Autodesk Inventor part; units mm, degrees
ref_plane "YZ Plane" through (0, 0, 0) normal (1, 0, 0) x (0, 1, 0)
ref_plane "XZ Plane" through (0, 0, 0) normal (0, 1, 0) x (-1, 0, 0)
ref_plane "XY Plane" through (0, 0, 0) normal (0, 0, 1) x (1, 0, 0)
sketch "Szkic1" plane through (0, 0, 0) normal (0, 1, 0) x (-1, 0, 0)
  line L0 (28, 0) -> (0, 0)
  line L1 (0, 0) -> (0, -8)
  line L2 (0, -8) -> (28, -8)
  line L3 (28, -8) -> (28, 0)
  dimension "d0" = 8
  dimension "d4" = 28
extrude "Wyciągnięcie proste1" add sketch "Szkic1" along normal blind 2.5
sketch "Szkic2" plane through (0, 2.5, 0) normal (0, 1, 0) x (1, 0, 0)
  line L0 (-28, 0) -> (0, 0)
  line L1 (0, 8) -> (-28, 8)
  line L2 (-14, 0) -> (-14, 8)
  line L3 (-24, 4) -> (-4, 4)
  point P0 (-14, 4)
  dimension "d3" = 20
hole "Otwór1" at (-24, 2.5, -4) at (-4, 2.5, -4) direction (0, -1, 0) diameter 2.6 end through all counterbore diameter 4.5 counterbore depth 1.5
sketch "Szkic3" plane through (-28, 0, 0) normal (0, 0, 1) x (1, 0, 0)
  line L0 (14, 2.5) -> (14, 0)
  line L1 (0, 2.5) -> (28, 2.5)
  line L2 (0, 0) -> (28, 0)
  circle A0 centre (14, -5) radius 2.5
  line L3 (10, -5) -> (18, -5)
  line L4 (18, -5) -> (18, 0)
  line L5 (10, 0) -> (10, -5)
  line L6 (18, 0) -> (10, 0)
  point P0 (10, 3)
  point P1 (17.6174, 3)
  point P2 (16.5, -5)
  point P3 (11.5, -5)
  point P4 (14, 0)
  point P5 (18, 0)
  dimension "d12" = 5
  dimension "d13" = 8
  dimension "d17" = 5
extrude "Wyciągnięcie proste2" add sketch "Szkic3" against normal up to surface (8 mm away) contours L2 L4 L3 A0 L5
fillet "Zaokrąglenie1" radius 2 4 edges at (0, 1.25, 0) (0, 1.25, -8) (-28, 1.25, -8) (-28, 1.25, 0)
equation "\"d0\" = obudowa_led_mocowanie_grubosc"
equation "\"d4\" = holder_led_dlugosc"
equation "\"d1\" = holder_led_grubosc"
equation "\"d5\" = gniazdo_M2_D2"
equation "\"d7\" = gniazdo_M2_D1"
equation "\"d8\" = gniazdo_M2_glebokosc"
equation "\"d10\" = insert_glebokosc"
equation "\"d12\" = holder_led_uchwyt_D"
equation "\"d13\" = holder_led_uchwyt_szerokosc"
equation "\"d17\" = holder_led_uchwyt_wysokosc"
equation "\"gniazdo_M2_glebokosc\" = 1.5"
equation "\"gniazdo_M2_D1\" = 4.5"
equation "\"gniazdo_M2_D2\" = 2.6"
equation "\"insert_D\" = 2.9"
equation "\"insert_glebokosc\" = 7"
equation "\"podstawa_wys\" = 2"
equation "\"podstawa_otwory_montazowe_poz_x\" = 4"
equation "\"podstawa_otwory_montazowe_poz_y\" = 4"
equation "\"podstawa_zaokraglenie\" = 3"
equation "\"obudowa_wys\" = 45"
equation "\"obudowa_grubosc\" = 2"
equation "\"obudowa_kontrolki_a\" = 38"
equation "\"obudowa_otwory_montazowe_poz_x\" = 4"
equation "\"obudowa_otwory_montazowe_poz_y\" = 4"
equation "\"obudowa_otwory_montazowe_material_x\" = 8"
equation "\"obudowa_otwory_montazowe_material_y\" = 8"
equation "\"obudowa_zaokraglenie\" = 3"
equation "\"obudowa_otwory_io1_D\" = 12"
equation "\"obudowa_otwory_io1_wys\" = 25"
equation "\"obudowa_otwory_io1_poz\" = 55"
equation "\"obudowa_otwory_io2_D\" = 12"
equation "\"obudowa_otwory_io2_wys\" = 25"
equation "\"obudowa_otwory_io2_poz\" = 38"
equation "\"obudowa_otwory_pot_D\" = 7.2"
equation "\"obudowa_pot_poz_y\" = 15"
equation "\"obudowa_s_rozstaw_y\" = 16"
equation "\"obudowa_s_poz_x\" = 78"
equation "\"obudowa_s_poz_y\" = 15"
equation "\"obudowa_s_D\" = 6.2"
equation "\"input_a\" = 8.9"
equation "\"input_b\" = 14.4"
equation "\"input_wys\" = 10.9"
equation "\"obudowa_MTS_otwor_D\" = 6.2"
equation "\"pcb_rozstaw_x\" = 92"
equation "\"pcb_rozstaw_y\" = 58"
equation "\"pcb_grubosc_scianki\" = 6"
equation "\"pcb_wys_bloku\" = 35"
equation "\"pcb_poz_y\" = 29"
equation "\"obudowa_footswitch_D\" = 12.3"
equation "\"obudowa_footswitch_poz_x\" = 35"
equation "\"obudowa_footswitch_poz_y\" = 68"
equation "\"obudowa_led_indicator_D\" = 3.5"
equation "\"obudowa_led_indicator_poz_x\" = 55"
equation "\"obudowa_podkladka_otwory\" = 4"
equation "\"obudowa_uchwyt_poz_z\" = 3"
equation "\"obudowa_uchwyt_grubosc\" = 2"
equation "\"obudowa_uchwyt_szerokosc_wew\" = 17.5"
equation "\"obudowa_uchwyt_wysokosc_wew\" = 26.3"
equation "\"obudowa_uchwyt_kolnierz_wys\" = 55"
equation "\"obudowa_gniazdo_poz\" = 25"
equation "\"obudowa_podciecie_inout_wys\" = 6"
equation "\"obudowa_podciecie_logo_wys\" = 34"
equation "\"obudowa_podciecie_logo_szerokosc\" = 25"
equation "\"obudowa_pot_pozycjonowanie_szerokosc\" = 2.8"
equation "\"obudowa_pot_pozycjonowanie_wys\" = 13"
equation "\"obudowa_pot_pozycjonowanie_glebokosc\" = 1.4"
equation "\"obudowa_led_mocowanie_wys\" = 6"
equation "\"obudowa_led_mocowanie_grubosc\" = 8"
equation "\"obudowa_led_mocowanie_rozstaw_otworow\" = 20"
equation "\"holder_led_grubosc\" = 2.5"
equation "\"holder_led_dlugosc\" = 28"
equation "\"holder_led_uchwyt_D\" = 5"
equation "\"holder_led_uchwyt_wysokosc\" = 5"
equation "\"holder_led_uchwyt_szerokosc\" = 8"
equation "\"holder_gniazdo_b\" = 5"
equation "\"holder_gniazdo_grubosc\" = 2.5"
equation "\"holder_gniazdo_a\" = 28"
equation "\"podstawa_mocowanie_DC_a\" = 7"
equation "\"podstawa_mocowanie_DC_b\" = 8.9"
equation "\"podstawa_mocowanie_DC_wys\" = 6"
equation "\"holder_gniazdo_odleglosc_miedzy_ramionami\" = 9.2"
equation "\"holder_gniazdo_grubosc_ramion\" = 1.5"
equation "\"holder_gniazdo_wys\" = 8"
equation "\"holder_gniazdo_uchwyt_poz\" = 5"
properties part number "led_holder"
Here's how the part is built. I have some questions about the finished solid (model axes, mm). A direction names the side the tool comes from. Round coordinates to 2 decimals unless told otherwise and drop trailing zeros. Loops run counter-clockwise (first coordinate to the right, second up) from the corner with the lowest first, then second, coordinate; pieces in that order, holes last. Notation, with made-up numbers: (-17.75, -14.5) -> (31.25, -14.5) arc R24 ccw to (31.25, 20.5) -> close; hole circle Ø11 at (44.5, -34.5). An arc over 180 degrees is marked (long way). Write each question's results on one line, items separated by ' | '.
(1) If we section it at B-B, the plane x = -24: List the corners of the cut face in (y, z) for me.
Worked answers:
outline: (0, -8) -> (2.5, -8) -> (2.5, -6.25) -> (1, -6.25) -> (1, -5.3) -> (0, -5.3) -> close; (0, -2.7) -> (1, -2.7) -> (1, -1.75) -> (2.5, -1.75) -> (2.5, 0) -> (0, 0) -> close
(2) If we section it at A-A, the plane y = -3.5: List the corners of the cut face in (x, z) for me, then the cut area to 3 significant figures.
Worked answers:
outline: (-18, -8) -> (-16, -8) -> (-16, 0) -> (-18, 0) -> close; (-12, -8) -> (-10, -8) -> (-10, 0) -> (-12, 0) -> close | area: 32.0 mm2
(3) If I drill on L1, parallel to X at y = 2.05, z = -4; L2, parallel to X at y = 0.45, z = -4; L3, parallel to Z at x = -24, y = 0.65, over which ranges is the centre line in solid material (lowest first)?
Worked answers:
L1: -28 to -26.25, -21.75 to -6.25, -1.75 to 0 | L2: -28 to -25.3, -22.7 to -5.3, -2.7 to 0 | L3: -8 to -5.3, -2.7 to 0
(4) We'd pull the mould along X, two halves only. Please class faces 4 (the face through (-13.9, -2.5, -3.9)), 5 (the face through (-14, 0, -8)), 6 (the face through (-27.43, 1.27, -0.6)), 7 (the face through (-0.57, 1.27, -7.4)): released by +X, released by -X, zero draft, split by the parting line, or undercut.
Worked answers:
face 4: undercut | face 5: zero draft | face 6: released by -X | face 7: released by +X
(5) For faces 1 (the face through (-24, 1, -2.5)), 2 (the face through (-10, -3, -4)), 3 (the face through (-18, -2, -4)), which set-ups out of +Z, -Z, +X, -X, +Y, -Y let a thin tool reach every point of the face, with its end or its side?
Worked answers:
face 1: +Y | face 2: +Z, -Z, +X, -Y | face 3: +Z, -Z, -X, -Y
(6) If we section it at D-D, the plane y = 1.75: List the corners of the cut face in (x, z) for me, then the cut area to 3 significant figures.
Worked answers:
outline: (-28, -6) arc R2 ccw to (-26, -8) -> (-2, -8) arc R2 ccw to (0, -6) -> (0, -2) arc R2 ccw to (-2, 0) -> (-26, 0) arc R2 ccw to (-28, -2) -> close; hole circle Ø4.5 at (-24, -4); hole circle Ø4.5 at (-4, -4) | area: 189 mm2
(7) For P1, Ø1.5, axis at y = -3.5, z = -5.5, coming from the +X side; P2, Ø1.5, axis at y = -3, z = -3.5, coming from the -X side; P3, Ø1.3, axis at x = -23.5, z = -3, coming from the +Y side, each with a flat end and sliding along its axis, tell me the tip position at first contact or that it passes through.
Worked answers:
P1: x = -10 | P2: x = -18 | P3: y = 1
(8) If we section it at C-C, the plane z = -4: List the corners of the cut face in (x, y) for me.
Worked answers:
outline: (-28, 0) -> (-25.3, 0) -> (-25.3, 1) -> (-26.25, 1) -> (-26.25, 2.5) -> (-28, 2.5) -> close; (-22.7, 0) -> (-18, 0) -> (-18, -5) -> (-16.5, -5) arc R2.5 cw to (-11.5, -5) -> (-10, -5) -> (-10, 0) -> (-5.3, 0) -> (-5.3, 1) -> (-6.25, 1) -> (-6.25, 2.5) -> (-21.75, 2.5) -> (-21.75, 1) -> (-22.7, 1) -> close; (-2.7, 0) -> (0, 0) -> (0, 2.5) -> (-1.75, 2.5) -> (-1.75, 1) -> (-2.7, 1) -> close
